Design review of the part shown in the three views and the two pictorial views. Dimensions are in mm from the part's minimum x, y and z. A direction names the side the tool comes from. Coordinates: 2 decimals unless noted, no trailing zeros. Loops run counter-clockwise (first coordinate to the right, second up) from the corner with the lowest first, then second, coordinate; pieces in that order, holes last. Notation, with made-up numbers: (-26, 62.5) -> (-20, 62.5) arc R18 cw to (-20, 96.5) -> close; hole circle Ø8 at (1.5, 61). An arc over 180 degrees is marked (long way). Use a Markdown table: item, result. Add a question column.
Q1. Take a section at B-B on y = 21. Write out the cut boundary in (x, z), plus the area to 3 significant figures.
Q2. For probe 1 along Y at (x, z) = (21, 33); probe 2 along Z at (x, y) = (38.5, 4); probe 3 along Y at (x, z) = (9, 5), list the stretches that pass through material, from the lowest coordinate up.
Q3. Take a section at D-D on z = 16. Write out the cut boundary in (x, y), plus the area to 3 significant figures.
Q4. For the marked faces 1, 2, 3 and 4, list the 3-axis set-ups (+Z, -Z, +X, -X, +Y, -Y) from which the entire face can be reached by the end or side of a thin tool; tool diameter is ignored.
Q5. Take a section at A-A on z = 7. Write out the cut boundary in (x, y).
Q6. Take a section at C-C on x = 21. Write out the cut boundary in (y, z).
Q7. Clearance check with flat-ended pins moving along their axes: pin 1 Ø3 at (x, y) = (14, 11) entering from +Z; pin 2 Ø6 at (x, y) = (20.5, 45.5) entering from +Z; pin 3 Ø1 at (x, y) = (18, 9) entering from +Z. State where each tip first meets the part, or that it passes through.
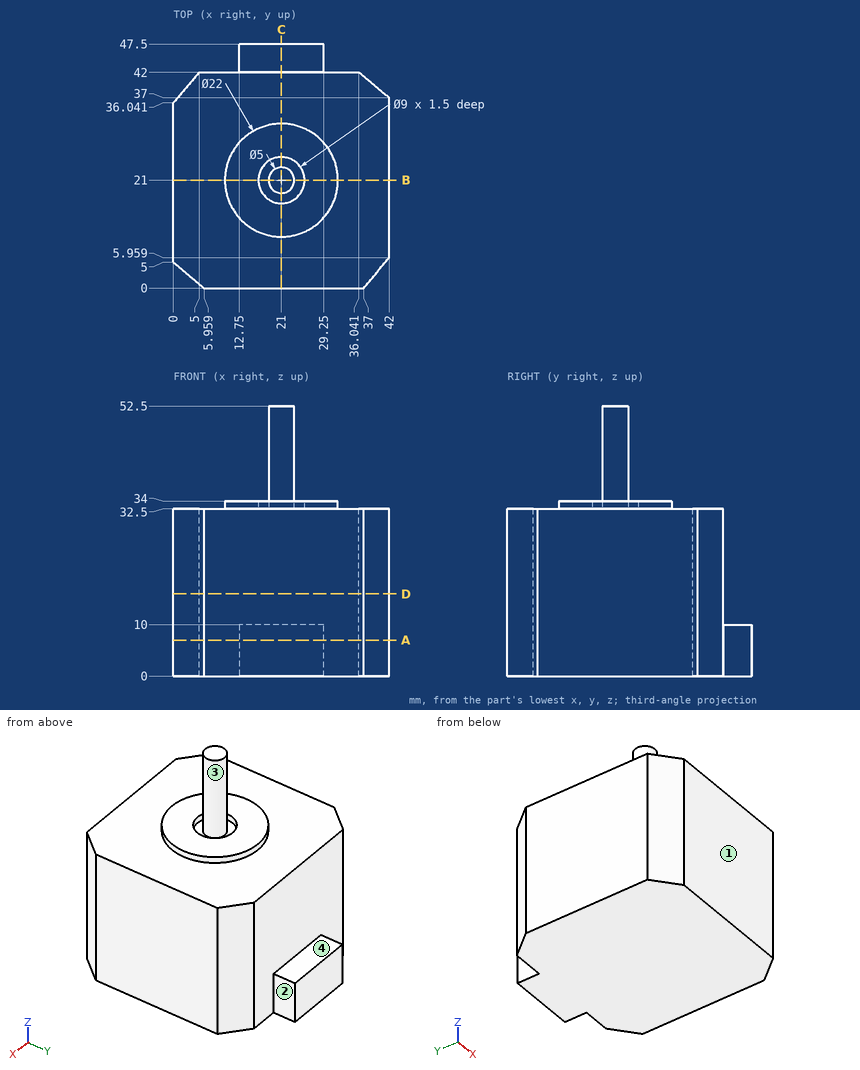
Answer list:
| question | item | result |
|---|---|---|
| 1 | outline | (0, 0) -> (42, 0) -> (42, 32.5) -> (32, 32.5) -> (32, 34) -> (25.5, 34) -> (25.5, 32.5) -> (23.5, 32.5) -> (23.5, 52.5) -> (18.5, 52.5) -> (18.5, 32.5) -> (16.5, 32.5) -> (16.5, 34) -> (10, 34) -> (10, 32.5) -> (0, 32.5) -> close |
| 1 | area | 1,480 mm² |
| 2 | probe 1 | 10 to 16.5, 18.5 to 23.5, 25.5 to 32 |
| 2 | probe 2 | 0 to 32.5 |
| 2 | probe 3 | 0 to 42 |
| 3 | outline | (0, 5) -> (5.96, 0) -> (37, 0) -> (42, 5.96) -> (42, 37) -> (36.04, 42) -> (5, 42) -> (0, 36.04) -> close |
| 3 | area | 1,700 mm² |
| 4 | face 1 | +Z, -Z, +X, -X, -Y |
| 4 | face 2 | +Z, -Z, +X, +Y |
| 4 | face 3 | +Z |
| 4 | face 4 | +Z, +X, -X, +Y |
| 5 | outline | (0, 5) -> (5.96, 0) -> (37, 0) -> (42, 5.96) -> (42, 37) -> (36.04, 42) -> (29.25, 42) -> (29.25, 47.5) -> (12.75, 47.5) -> (12.75, 42) -> (5, 42) -> (0, 36.04) -> close |
| 6 | outline | (0, 0) -> (47.5, 0) -> (47.5, 10) -> (42, 10) -> (42, 32.5) -> (32, 32.5) -> (32, 34) -> (25.5, 34) -> (25.5, 32.5) -> (23.5, 32.5) -> (23.5, 52.5) -> (18.5, 52.5) -> (18.5, 32.5) -> (16.5, 32.5) -> (16.5, 34) -> (10, 34) -> (10, 32.5) -> (0, 32.5) -> close |
| 7 | pin 1 | z = 34 |
| 7 | pin 2 | z = 10 |
| 7 | pin 3 | z = 32.5 |
